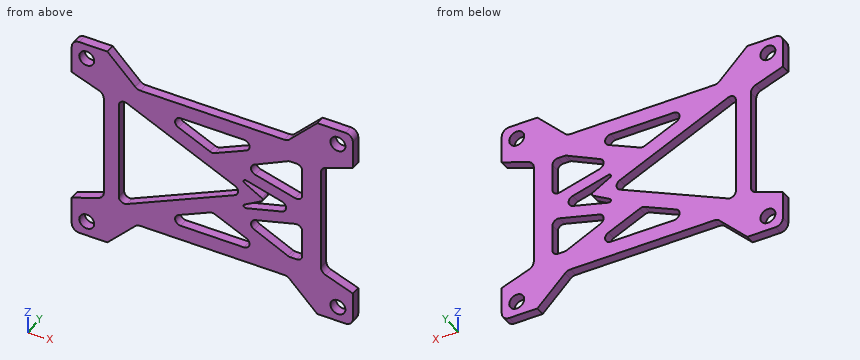
```python
from build123d import *

# Parameters (mm, degrees)
EXTRUDE_1_DEPTH     = 2.5
FILLET_2_R          = 1.5
FILLET_3_R          = 0.5
SKETCH_3_R          = 2
CUT_EXTRUDE_1_DEPTH = 47.569840025
FILLET_4_R          = 2


with BuildPart() as part:
    # 草图2 → 凸台-拉伸1 (new body)
    with BuildSketch(Plane(origin=(0, 0, 0), x_dir=(1, 0, 0), z_dir=(0, 1, 0))):
        Polygon((-37.5, 27.5), (-28, 27.5), (-20, 19.5), (20, 19.5), (28, 27.5), (37.5, 27.5), (37.5, 18.111945503), (28.95, 15), (28.95, -15), (37.5, -18.111945503), (37.5, -27.5), (28, -27.5), (20, -19.5), (-20, -19.5), (-28, -27.5), (-37.5, -27.5), (-37.5, -18.111945503), (-28.95, -15), (-28.95, 15), (-37.5, 18.111945503), align=None)
        Polygon((15.323396198, 15.5), (0, 8.5), (-15.323396198, 15.5), align=None, mode=Mode.SUBTRACT)
        Polygon((-24.95, 15.5), (-24.95, -15.5), (8.980377297, 0), align=None, mode=Mode.SUBTRACT)
        Polygon((-15.323396198, -15.5), (15.323396198, -15.5), (0, -8.5), align=None, mode=Mode.SUBTRACT)
        Polygon((5.320123259, 5), (13.980377297, 0), (5.320123259, -5), (23.980377297, 0), align=None, mode=Mode.SUBTRACT)
        Polygon((7.499709521, 7.581961581), (20.478475988, 13.793792116), (23.980377297, 13.793792116), (23.980377297, 3.206634177), align=None, mode=Mode.SUBTRACT)
        Polygon((23.980377297, -13.793792116), (23.980377297, -3.206634177), (7.499709521, -7.581961581), (20.478475988, -13.793792116), align=None, mode=Mode.SUBTRACT)
    extrude(amount=EXTRUDE_1_DEPTH)

    # 圆角2
    fillet_2_edges = [part.edges().sort_by_distance(p)[0] for p in [
        (20.478475988, 1.25, 13.793792116),
        (23.980377297, 1.25, 13.793792116),
        (23.980377297, 1.25, 3.206634177),
        (7.499709521, 1.25, 7.581961581),
        (0, 1.25, 8.5),
        (-15.323396198, 1.25, 15.5),
        (15.323396198, 1.25, 15.5),
        (8.980377297, 1.25, 0),
        (-24.95, 1.25, -15.5),
        (-24.95, 1.25, 15.5),
        (-15.323396198, 1.25, -15.5),
        (0, 1.25, -8.5),
        (15.323396198, 1.25, -15.5),
        (23.980377297, 1.25, 0),
        (7.499709521, 1.25, -7.581961581),
        (23.980377297, 1.25, -3.206634177),
        (23.980377297, 1.25, -13.793792116),
        (20.478475988, 1.25, -13.793792116),
    ]]
    fillet(fillet_2_edges, radius=FILLET_2_R)

    # 圆角3
    fillet_3_edges = [part.edges().sort_by_distance(p)[0] for p in [
        (5.320123259, 1.25, -5),
        (13.980377297, 1.25, 0),
        (5.320123259, 1.25, 5),
    ]]
    fillet(fillet_3_edges, radius=FILLET_3_R)

    # 草图3 → 切除-拉伸1 (cut, through all)
    with BuildSketch(Plane(origin=(0, 2.5, 0), x_dir=(1, 0, 0), z_dir=(0, 1, 0))):
        with Locations(Location((-33.5, -23.5, 0), (0, 0, 270))):
            Circle(SKETCH_3_R)
        with Locations(Location((33.5, -23.5, 0), (0, 0, 270))):
            Circle(SKETCH_3_R)
        with Locations(Location((33.5, 23.5, 0), (0, 0, 90))):
            Circle(SKETCH_3_R)
        with Locations(Location((-33.5, 23.5, 0), (0, 0, 90))):
            Circle(SKETCH_3_R)
    extrude(amount=-CUT_EXTRUDE_1_DEPTH, mode=Mode.SUBTRACT)

    # 圆角4
    fillet_4_edges = [part.edges().sort_by_distance(p)[0] for p in [
        (20, 1.25, 19.5),
        (-20, 1.25, 19.5),
        (-37.5, 1.25, 27.5),
        (-28.95, 1.25, 15),
        (-28.95, 1.25, -15),
        (-37.5, 1.25, -27.5),
        (-20, 1.25, -19.5),
        (20, 1.25, -19.5),
        (37.5, 1.25, -27.5),
        (28.95, 1.25, -15),
        (28.95, 1.25, 15),
        (37.5, 1.25, 27.5),
    ]]
    fillet(fillet_4_edges, radius=FILLET_4_R)


solid = part.part
```
Verification items for the finished model (mm, model axes). Give positions to 0.01 mm unless a question says otherwise; leave off trailing zeros. Order: outer loops, then holes, each group sorted by start corner. A loop starts at its lowest first (then second) coordinate and runs counter-clockwise, first axis right, second up. Notation, with made-up numbers: (7, 83) -> (59, 83) arc R19 ccw to (59, 91) -> close; hole circle Ø2 at (64, 79.5). An arc over 180 degrees is marked (long way). One line per item, written item: value.
(1) Sectioned sample at B-B on x = 16. Record the cut outline in (y, z).
Final values:
outline: (0, -19.5) -> (2.5, -19.5) -> (2.5, -11.65) -> (0, -11.65) -> close; (0, -5.33) -> (2.5, -5.33) -> (2.5, -2.14) -> (0, -2.14) -> close; (0, 2.14) -> (2.5, 2.14) -> (2.5, 5.33) -> (0, 5.33) -> close; (0, 11.65) -> (2.5, 11.65) -> (2.5, 19.5) -> (0, 19.5) -> close
(2) Sectioned sample at C-C on x = -16.5. Record the cut outline in (y, z), then the cut area to 3 significant figures.
Final values:
outline: (0, -19.5) -> (2.5, -19.5) -> (2.5, -11.64) -> (0, -11.64) -> close; (0, 11.64) -> (2.5, 11.64) -> (2.5, 19.5) -> (0, 19.5) -> close
area: 39.3 mm^2
(3) Gauge pin test, flat ends, axial feed: pin 1 (1.2 mm diameter, centred on y = 1.5, z = 3, fed in from +X); pin 2 (1.2 mm diameter, centred on x = 0.5, y = 1, fed in from -Z); pin 3 (1.5 mm diameter, centred on x = 2.5, y = 1.5, fed in from +Z); pin 4 (3 mm diameter, centred on x = 33.5, z = -23.5, fed in from -Y). Record the tip position at first contact, or that the pin passes through.
Final values:
pin 1: x = 28.95
pin 2: z = -19.5
pin 3: z = 19.5
pin 4: through
(4) Scan lines: line 1 along X through (y, z) = (0.5, -23.5); line 2 along Z through (x, y) = (-33, 0.9); line 3 along Z through (x, y) = (-11.5, 1.6). Record each from-to range of solid material in increasing order. Write a range as [from, to].
Final values:
line 1: [-37.5, -35.5], [-31.5, -24], [24, 31.5], [35.5, 37.5]
line 2: [-27.5, -25.44], [-21.56, -16.47], [16.47, 21.56], [25.44, 27.5]
line 3: [-19.5, -9.36], [9.36, 19.5]
(5) Sectioned sample at A-A on z = 23.5. Record the cut outline in (x, y), then the cut area to 3 significant figures.
Final values:
outline: (-37.5, 0) -> (-35.5, 0) -> (-35.5, 2.5) -> (-37.5, 2.5) -> close; (-31.5, 0) -> (-24, 0) -> (-24, 2.5) -> (-31.5, 2.5) -> close; (24, 0) -> (31.5, 0) -> (31.5, 2.5) -> (24, 2.5) -> close; (35.5, 0) -> (37.5, 0) -> (37.5, 2.5) -> (35.5, 2.5) -> close
area: 47.5 mm^2
(6) Sectioned sample at D-D on z = 7.5. Record the cut outline in (x, y).
Final values:
outline: (-28.95, 0) -> (-24.95, 0) -> (-24.95, 2.5) -> (-28.95, 2.5) -> close; (-7.44, 0) -> (10.4, 0) -> (10.4, 2.5) -> (-7.44, 2.5) -> close; (23.98, 0) -> (28.95, 0) -> (28.95, 2.5) -> (23.98, 2.5) -> close
